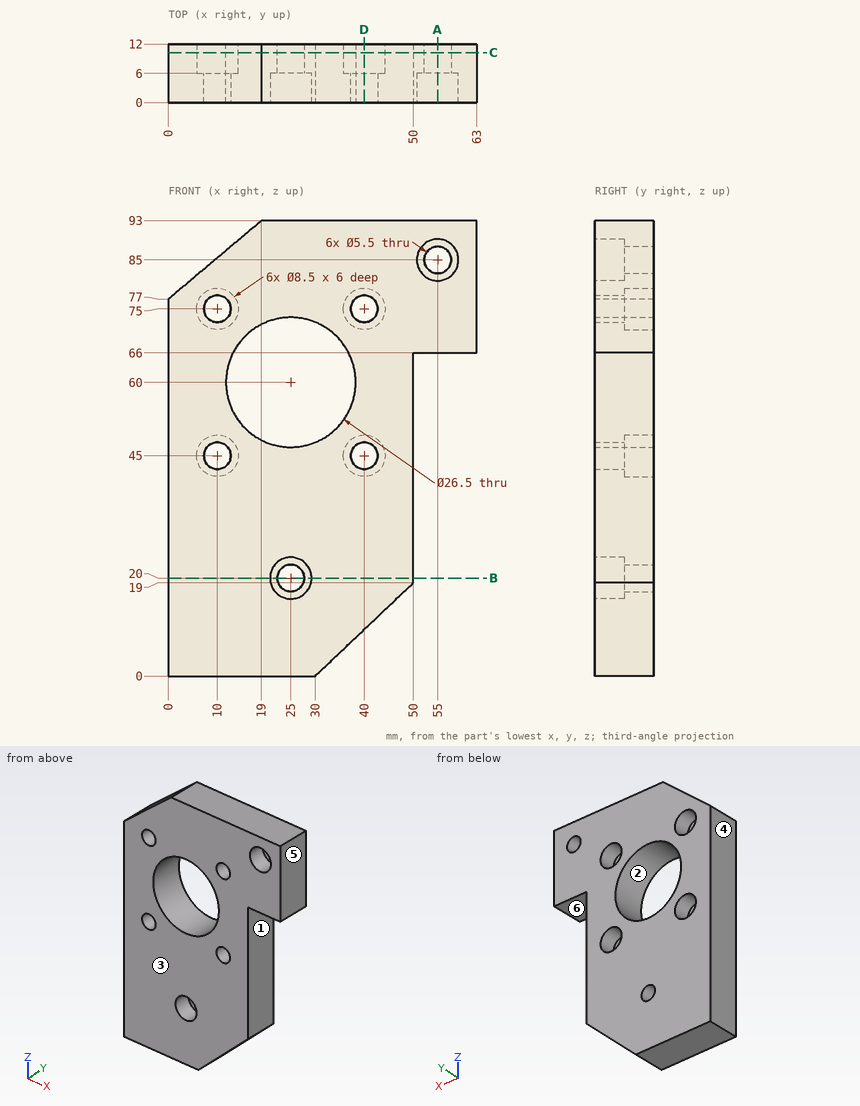
The figure shows three views and two pictorial views of one solid part (mm, origin at its lowest corner). Answer the questions. A direction names the side the tool comes from. Round coordinates to 2 decimals unless told otherwise and drop trailing zeros. Loops run counter-clockwise (first coordinate to the right, second up) from the corner with the lowest first, then second, coordinate; pieces in that order, holes last. Notation, with made-up numbers: M 71.5,-12 L 89.5,-12 A29 ccw 89.5,19 Z; hole C -17.5,-10.5 d5. An arc over 180 degrees is marked long. Write each question's results on one line, items separated by ' | '. Start each with the question number.
1) Find section A-A on x = 55. Write down the section's boundary in (y, z), plus the area to 3 significant figures.
2) Each of these flat-tipped pins is pushed along its axis until it touches: pin 1 (9.5 mm diameter, centred on x = 40, z = 74.5, fed in from +Y); pin 2 (1.5 mm diameter, centred on y = 2, z = 36.5, fed in from +X); pin 3 (6.5 mm diameter, centred on x = 25, z = 20, fed in from -Y); pin 4 (4 mm diameter, centred on x = 9, z = 44.5, fed in from +Y). Where does it stop, or does it pass through?
3) Find section C-C on y = 10.25. Write down the section's boundary in (x, z), plus the area to 3 significant figures.
4) Determine the mould class of the marked faces 1, 2, 3 and 4 for opening direction X: pulls with the +X half, pulls with the -X half, needs draft (parallel to the pull), parting line crosses it, or undercut.
5) Straight lines are drawn through the part: probe 1 along Z at (x, y) = (25, 4.75); probe 2 along X at (y, z) = (3.5, 75); probe 3 along Z at (x, y) = (25, 7.25). For each, find the intervals that lie inside material, in ascending order.
6) Which of the six approach directions +Z, -Z, +X, -X, +Y, -Y give full straight-line access (tool end or side, diameter ignored) to the marked faces 5 and 6?
7) Find section D-D on x = 40. Write down the section's boundary in (y, z).
8) Find section B-B on z = 20. Write down the section's boundary in (x, y), plus the area to 3 significant figures.
Final values:
1) outline: M 0,66 L 12,66 L 12,82.25 L 6,82.25 L 6,80.75 L 0,80.75 Z; M 0,89.25 L 6,89.25 L 6,87.75 L 12,87.75 L 12,93 L 0,93 Z | area: 240 mm²
2) pin 1: y = 12 | pin 2: x = 50 | pin 3: y = 6 | pin 4: y = 6
3) outline: M 0,0 L 30,0 L 50,19 L 50,66 L 63,66 L 63,93 L 19,93 L 0,77 Z; hole C 10,45 d8.5; hole C 10,75 d8.5; hole C 25,60 d26.5; hole C 25,20 d5.5; hole C 40,45 d8.5; hole C 40,75 d8.5; hole C 55,85 d5.5 | area: 3,830 mm²
4) face 1: pulls with the +X half | face 2: undercut | face 3: needs draft | face 4: pulls with the -X half
5) probe 1: 0 to 15.75, 24.25 to 46.75, 73.25 to 93 | probe 2: 0 to 7.25, 12.75 to 37.25, 42.75 to 63 | probe 3: 0 to 17.25, 22.75 to 46.75, 73.25 to 93
6) face 5: +Z, -Z, +X, +Y, -Y | face 6: -Z, +X, +Y, -Y
7) outline: M 0,9.5 L 12,9.5 L 12,40.75 L 6,40.75 L 6,42.25 L 0,42.25 Z; M 0,47.75 L 6,47.75 L 6,49.25 L 12,49.25 L 12,70.75 L 6,70.75 L 6,72.25 L 0,72.25 Z; M 0,77.75 L 6,77.75 L 6,79.25 L 12,79.25 L 12,93 L 0,93 Z
8) outline: M 0,0 L 20.75,0 L 20.75,6 L 22.25,6 L 22.25,12 L 0,12 Z; M 27.75,6 L 29.25,6 L 29.25,0 L 50,0 L 50,12 L 27.75,12 Z | area: 516 mm²
